from build123d import *

# Parameters (mm, degrees)
SKETCH2_W           = 38.1
SKETCH2_H           = 76.2
BOSS_EXTRUDE1_DEPTH = 12.7
SKETCH3_R           = 1.905
BOSS_EXTRUDE3_DEPTH = 11.43
SKETCH5_W           = 38.1
SKETCH5_H           = 18.614666354
BOSS_EXTRUDE5_DEPTH = 2.54
SKETCH6_W           = 38.1
SKETCH6_H           = 18.614666354
BOSS_EXTRUDE6_DEPTH = 3.81


with BuildPart() as part:
    # Sketch2 → Boss-Extrude1 (new body)
    with BuildSketch(Plane(origin=(0, 0, 0), x_dir=(1, 0, 0), z_dir=(0, 1, 0))):
        with Locations((19.05, 38.1)):
            Rectangle(SKETCH2_W, SKETCH2_H)
    extrude(amount=BOSS_EXTRUDE1_DEPTH)

    # Sketch3 → Boss-Extrude3 (add)
    with BuildSketch(Plane.ZY):
        with Locations(Location((-25.4, 6.478602977, 0), (0, 0, 180))):
            Circle(SKETCH3_R)
    extrude(amount=BOSS_EXTRUDE3_DEPTH)

    # Sketch5 → Boss-Extrude5 (add)
    with BuildSketch(Plane(origin=(0, 12.7, 0), x_dir=(1, 0, 0), z_dir=(0, 1, 0))):
        with Locations((19.05, 9.307333177)):
            Rectangle(SKETCH5_W, SKETCH5_H)
    extrude(amount=BOSS_EXTRUDE5_DEPTH)

    # Sketch6 → Boss-Extrude6 (add)
    with BuildSketch(Plane(origin=(0, 15.24, 0), x_dir=(1, 0, 0), z_dir=(0, 1, 0))):
        with Locations((19.05, 9.307333177)):
            Rectangle(SKETCH6_W, SKETCH6_H)
    extrude(amount=BOSS_EXTRUDE6_DEPTH)


solid = part.part
Design review of the part built by this model. Coordinates are the model's own, in mm. A direction names the side the tool comes from. Give positions to 0.01 mm unless a question says otherwise; leave off trailing zeros. Loops run counter-clockwise (first coordinate to the right, second up) from the corner with the lowest first, then second, coordinate; pieces in that order, holes last. Notation, with made-up numbers: M 43.25,34.5 L 55.25,34.5 A14 ccw 55.25,54.5 Z; hole C -4.5,-1 d4. An arc over 180 degrees is marked long. Write item = value, one per line.
Q1. For faces 1 (the cylindrical face through (-5.635, 6.395, -23.497)), 2 (the flat face through (19, 0, -39)), 3 (the flat face through (19, 16, -18.615)), list the 3-axis set-ups (+Z, -Z, +X, -X, +Y, -Y) from which the entire face can be reached by the end or side of a thin tool; tool diameter is ignored.
Output values:
face_1 = -X
face_2 = +Z, -Z, +X, -X, -Y
face_3 = -Z, +X, -X, +Y
Q2. To check wall thickness, follow line 1 (Y direction, x = 23, z = -51.5); line 2 (X direction, y = 3.25, z = -13.5); line 3 (Z direction, x = 33, y = 17.5). State the ranges of each line that lie inside material, in increasing order. Write a range as [from, to].
Output values:
line_1 = [0, 12.7]
line_2 = [0, 38.1]
line_3 = [-18.61, 0]
Q3. Insertion check: pin 1 (5.5 mm diameter, centred on y = 8, z = -37, fed in from -X); pin 2 (6 mm diameter, centred on x = 17, z = -33.5, fed in from +Y). Each pin has a flat end and moves straight along its axis. Give the tip position at first contact, or say it passes through.
Output values:
pin_1 = 0
pin_2 = 12.7
Q4. We need section A-A (x = 14.5). Give the boundary of the cut face in (y, z), plus the area to 3 significant figures.
Output values:
outline = M 0,-76.2 L 12.7,-76.2 L 12.7,-18.61 L 19.05,-18.61 L 19.05,0 L 0,0 Z
area = 1,090 mm^2
Q5. We need section C-C (y = 15.5). Give the boundary of the cut face in (x, z), plus the area to 3 significant figures.
Output values:
outline = M 0,-18.61 L 38.1,-18.61 L 38.1,0 L 0,0 Z
area = 709 mm^2
Q6. We need section D-D (z = -42.5). Give the boundary of the cut face in (x, y), plus the area to 3 significant figures.
Output values:
outline = M 0,0 L 38.1,0 L 38.1,12.7 L 0,12.7 Z
area = 484 mm^2
Q7. We need section B-B (z = -25.4). Give the boundary of the cut face in (x, y).
Output values:
outline = M -11.43,4.57 L 0,4.57 L 0,0 L 38.1,0 L 38.1,12.7 L 0,12.7 L 0,8.38 L -11.43,8.38 Z
